Model file for the job. Use its own axes, mm. Round coordinates to 2 decimals unless told otherwise and drop trailing zeros. Loops run counter-clockwise (first coordinate to the right, second up) from the corner with the lowest first, then second, coordinate; pieces in that order, holes last. Notation, with made-up numbers: (36.25, 11) -> (60.25, 11) arc R30 ccw to (60.25, 34) -> close; hole circle Ø10 at (24.25, 26). An arc over 180 degrees is marked (long way). Use a Markdown table: item, result.
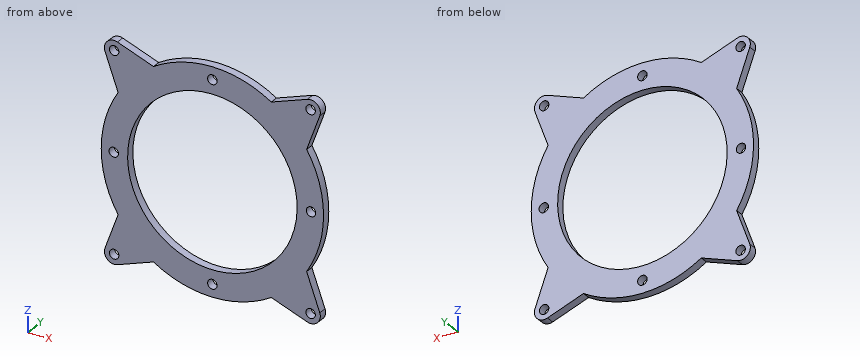
from build123d import *

# Parameters (mm, degrees)
SKETCH_1_R      = 30.5
SKETCH_1_R_2    = 1.7
EXTRUDE_1_DEPTH = 3


with BuildPart() as part:
    # 草图1 → 凸台-拉伸1 (new body)
    with BuildSketch(Plane(origin=(0, 0, 0), x_dir=(1, 0, 0), z_dir=(0, 1, 0))):
        with BuildLine():
            Line((34.158268558, 38.644263232), (21.19197667, 33.924918936))
            ThreePointArc((21.19197667, 33.924918936), (0, 40), (-21.19197667, 33.924918936))
            Line((-21.19197667, 33.924918936), (-34.158268558, 38.644263232))
            ThreePointArc((-34.158268558, 38.644263232), (-37.830212793, 37.830212793), (-38.644263232, 34.158268558))
            Line((-38.644263232, 34.158268558), (-33.924918936, 21.19197667))
            ThreePointArc((-33.924918936, 21.19197667), (-40, 0), (-33.924918936, -21.19197667))
            Line((-33.924918936, -21.19197667), (-38.644263232, -34.158268558))
            ThreePointArc((-38.644263232, -34.158268558), (-37.830212793, -37.830212793), (-34.158268558, -38.644263232))
            Line((-34.158268558, -38.644263232), (-21.19197667, -33.924918936))
            ThreePointArc((-21.19197667, -33.924918936), (0, -40), (21.19197667, -33.924918936))
            Line((21.19197667, -33.924918936), (34.158268558, -38.644263232))
            ThreePointArc((34.158268558, -38.644263232), (37.830212793, -37.830212793), (38.644263232, -34.158268558))
            Line((38.644263232, -34.158268558), (33.924918936, -21.19197667))
            ThreePointArc((33.924918936, -21.19197667), (40, 0), (33.924918936, 21.19197667))
            Line((33.924918936, 21.19197667), (38.644263232, 34.158268558))
            ThreePointArc((38.644263232, 34.158268558), (37.830212793, 37.830212793), (34.158268558, 38.644263232))
        make_face()
        with Locations(Location((0, 0, 0), (0, 0, 270))):
            Circle(SKETCH_1_R, mode=Mode.SUBTRACT)
        with Locations(Location((0, 35.5, 0), (0, 0, 270))):
            Circle(SKETCH_1_R_2, mode=Mode.SUBTRACT)
        with Locations(Location((35.5, 0, 0), (0, 0, 270))):
            Circle(SKETCH_1_R_2, mode=Mode.SUBTRACT)
        with Locations(Location((0, -35.5, 0), (0, 0, 270))):
            Circle(SKETCH_1_R_2, mode=Mode.SUBTRACT)
        with Locations(Location((-35.5, 0, 0), (0, 0, 270))):
            Circle(SKETCH_1_R_2, mode=Mode.SUBTRACT)
        with Locations(Location((35.355339059, 35.355339059, 0), (0, 0, 270))):
            Circle(SKETCH_1_R_2, mode=Mode.SUBTRACT)
        with Locations(Location((35.355339059, -35.355339059, 0), (0, 0, 270))):
            Circle(SKETCH_1_R_2, mode=Mode.SUBTRACT)
        with Locations(Location((-35.355339059, -35.355339059, 0), (0, 0, 270))):
            Circle(SKETCH_1_R_2, mode=Mode.SUBTRACT)
        with Locations(Location((-35.355339059, 35.355339059, 0), (0, 0, 270))):
            Circle(SKETCH_1_R_2, mode=Mode.SUBTRACT)
    extrude(amount=EXTRUDE_1_DEPTH)


solid = part.part
Q1. Drill centre lines: L1, parallel to Z at x = -25, y = 1.95; L2, parallel to Z at x = -20.5, y = 1.9; L3, parallel to X at y = 2.05, z = 23.5. Where is each one in solid material? Low to high. Write a range as from..to.
Results list:
| item | result |
|---|---|
| L1 | z = -35.31..-17.47, 17.47..35.31 |
| L2 | z = -34.35..-22.58, 22.58..34.35 |
| L3 | x = -34.76..-19.44, 19.44..34.76 |
Q2. Band-saw the part on A-A, the plane z = 0. Give the cut face in (x, y).
Results list:
| item | result |
|---|---|
| outline | (-40, 0) -> (-37.2, 0) -> (-37.2, 3) -> (-40, 3) -> close; (-33.8, 0) -> (-30.5, 0) -> (-30.5, 3) -> (-33.8, 3) -> close; (30.5, 0) -> (33.8, 0) -> (33.8, 3) -> (30.5, 3) -> close; (37.2, 0) -> (40, 0) -> (40, 3) -> (37.2, 3) -> close |
Q3. Band-saw the part on C-C, the plane z = 26.5. Give the cut face in (x, y), plus the area to 3 significant figures.
Results list:
| item | result |
|---|---|
| outline | (-35.86, 0) -> (-15.1, 0) -> (-15.1, 3) -> (-35.86, 3) -> close; (15.1, 0) -> (35.86, 0) -> (35.86, 3) -> (15.1, 3) -> close |
| area | 125 mm² |
Q4. Band-saw the part on D-D, the plane z = 35.5. Give the cut face in (x, y), plus the area to 3 significant figures.
Results list:
| item | result |
|---|---|
| outline | (-38.85, 0) -> (-37.05, 0) -> (-37.05, 3) -> (-38.85, 3) -> close; (-33.66, 0) -> (-25.52, 0) -> (-25.52, 3) -> (-33.66, 3) -> close; (-18.43, 0) -> (-1.7, 0) -> (-1.7, 3) -> (-18.43, 3) -> close; (1.7, 0) -> (18.43, 0) -> (18.43, 3) -> (1.7, 3) -> close; (25.52, 0) -> (33.66, 0) -> (33.66, 3) -> (25.52, 3) -> close; (37.05, 0) -> (38.85, 0) -> (38.85, 3) -> (37.05, 3) -> close |
| area | 160 mm² |
Q5. Band-saw the part on B-B, the plane x = -28. Give the cut face in (y, z), plus the area to 3 significant figures.
Results list:
| item | result |
|---|---|
| outline | (0, -36.4) -> (3, -36.4) -> (3, -12.09) -> (0, -12.09) -> close; (0, 12.09) -> (3, 12.09) -> (3, 36.4) -> (0, 36.4) -> close |
| area | 146 mm² |
Q6. Flat gauge pin, fed straight in: pin 1 (1.5 mm diameter, centred on y = 0.5, z = 31, fed in from +X). Where does the tip first touch, or does it go through?
Results list:
| item | result |
|---|---|
| pin 1 | stops at x = 37.77 |
